Geometry: final body of the model. Coordinates: model frame, mm. Give positions to 0.01 mm unless a question says otherwise; leave off trailing zeros. Write each loop counter-clockwise with the first axis right and the second up, starting at its lowest first coordinate (ties: lowest second). Pieces come first, ordered by that corner, then holes. Notation, with made-up numbers: (2.25, -36.75) - (35.25, -36.75) arc R18 cw to (35.25, -10.75) - close; hole circle Ø3 at (5.25, -13.75). An arc over 180 degrees is marked (long way). Use CSV: the item, a comma, the result in double quotes. Start each with the question number.
(1) First-contact query: pin 1 Ø12 at (x, z) = (-0.5, -48.5) entering from +Y; pin 2 Ø1 at (x, z) = (1, -16) entering from -Y; pin 3 Ø6 at (x, z) = (-0.5, 16) entering from +Y. Flat tips, straight axial feed; report the tip coordinate or a pass-through.
(2) Line query: probe 1 along Y at (x, z) = (6.5, -4); probe 2 along Y at (x, z) = (5, -40.5); probe 3 along X at (y, z) = (-59, 55.5). Output: solid intervals per line, ascending. Write a range as [from, to].
(3) Section B-B on x = -11. Output: boundary loops of the cut face in (y, z), and give its area (3 significant figures).
(4) Draft query along Y for faces 1 (the flat face through (-25, -610, -1)), 2 (the flat face through (12.675, -1181.481, 0.875)), 3 (the flat face through (-0.35, -30.21, 0.88)). Return one class per face: released by +Y, released by -Y, zero draft, split by the parting line, or undercut.
(5) Section A-A on z = 38. Output: boundary loops of the cut face in (x, y), and give its area (3 significant figures).
from build123d import *

# Parameters (mm, degrees)
F0_W     = 50
F0_H     = 125
F1_DEPTH = 1200
F3_DEPTH = 125
F5_DEPTH = 125


with BuildPart() as f1:
    # F0 (on Front) → F1 (new body)
    with BuildSketch(Plane.XZ):
        Rectangle(F0_W, F0_H)
    extrude(amount=F1_DEPTH)

    # F2 (on face) → F3 (cut, through all)
    with BuildSketch(Plane.XY.offset(62.5)):
        Polygon((-25, -59.58768), (25, 0), (-25, 0), align=None)
    extrude(amount=-F3_DEPTH, mode=Mode.SUBTRACT)

    # F4 (on face) → F5 (cut, through all)
    with BuildSketch(Plane.XY.offset(62.5)):
        Polygon((0, -1196.58671), (-25, -1175.609219), (-25, -1200), (25, -1200), (25, -1166.79287), align=None)
    extrude(amount=-F5_DEPTH, mode=Mode.SUBTRACT)


solid = f1.part
Check values:
1,pin 1,"stops at y = -23.24"
1,pin 2,"stops at y = -1195.99"
1,pin 3,"stops at y = -26.81"
2,probe 1,"y = [-1188.84, -22.05]"
2,probe 2,"y = [-1190.63, -23.84]"
2,probe 3,"x = [-24.51, 25]"
3,outline,"(-1187.36, -62.5) - (-42.9, -62.5) - (-42.9, 62.5) - (-1187.36, 62.5) - close"
3,area,"143,000 mm²"
4,face 1,"zero draft"
4,face 2,"released by -Y"
4,face 3,"released by +Y"
5,outline,"(-25, -1175.61) - (0, -1196.59) - (25, -1166.79) - (25, 0) - (-25, -59.59) - close"
5,area,"57,700 mm²"
